The figure shows three views and two pictorial views of one solid part (mm, origin at its lowest corner). Answer the questions. A direction names the side the tool comes from. Coordinates: 2 decimals unless noted, no trailing zeros. Loops run counter-clockwise (first coordinate to the right, second up) from the corner with the lowest first, then second, coordinate; pieces in that order, holes last. Notation, with made-up numbers: (44, 70) -> (48, 70) arc R25 ccw to (48, 104) -> close; hole circle Ø11 at (43.25, 49.5). An arc over 180 degrees is marked (long way). Use a Markdown table: item, result. Add a question column.
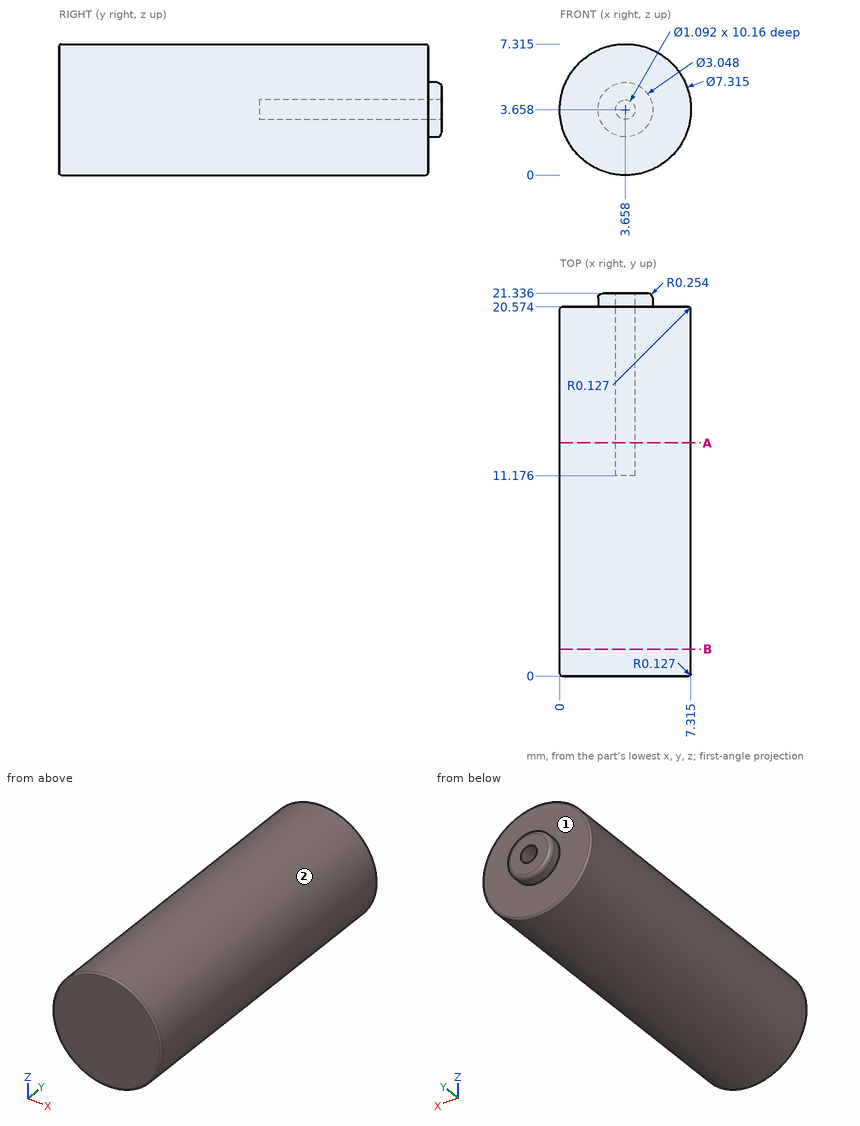
Item 1: Find the intervals of material crossed by probe 1 along Y at (x, z) = (2, 2.25); probe 2 along Z at (x, y) = (3.5, 8.5); probe 3 along X at (y, z) = (11.75, 3.5) (1 decimal), in increasing order.
Item 2: Section B-B (y = 1.5) is taken. Determine the outline of the cut face in (x, z) (1 decimal), then the cut area to 3 significant figures.
Item 3: Section A-A (y = 13) is taken. Determine the outline of the cut face in (x, z) (1 decimal), then the cut area to 3 significant figures.
Item 4: For the marked faces 1 and 2, determine the directions among +Z, -Z, +X, -X, +Y, -Y from which every point of the face is accessible in a straight line to the end or side of a thin tool.
Output:
| question | item | result |
|---|---|---|
| 1 | probe 1 | y = 0 to 20.57 |
| 1 | probe 2 | z = 0 to 7.31 |
| 1 | probe 3 | x = 0 to 3.1, 4.2 to 7.3 |
| 2 | outline | circle Ø7.3 at (3.7, 3.7) |
| 2 | area | 42.0 mm2 |
| 3 | outline | circle Ø7.3 at (3.7, 3.7); hole circle Ø1.1 at (3.7, 3.7) |
| 3 | area | 41.1 mm2 |
| 4 | face 1 | +Y |
| 4 | face 2 | +Y, -Y |
